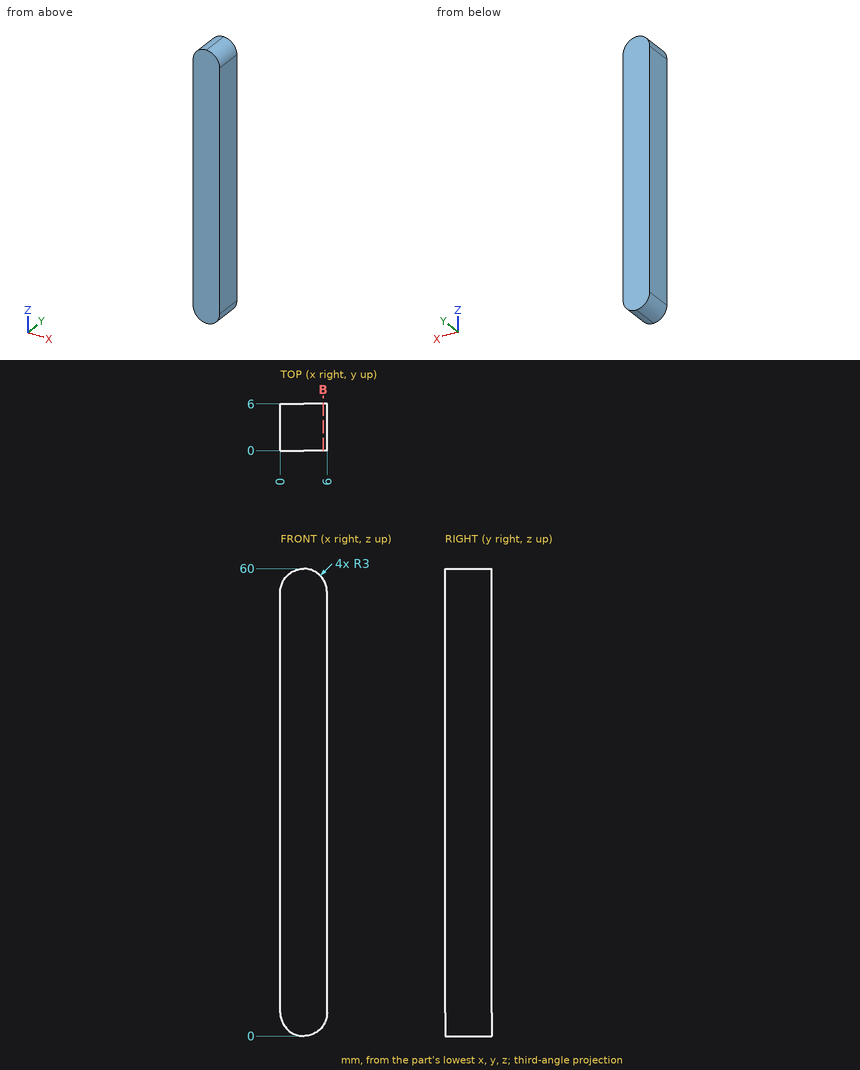
Could you check a few things on this drawing? It's one solid part, dimensions in mm from its lowest x, y, z. Coordinates: 2 decimals unless noted, no trailing zeros. Order: outer loops, then holes, each group sorted by start corner. A loop starts at its lowest first (then second) coordinate and runs counter-clockwise, first axis right, second up.
1) Imagine slicing it at B-B on x = 5.5. List the corners of the cut face in (y, z) for me, and give its area (3 significant figures).
2) I need wall thicknesses on line 1 (Z direction, x = 4.5, y = 3.4); line 2 (Z direction, x = 2, y = 1.6). Which ranges of each line are inside material? Lowest first, please.
3) Will this pin go through, and if not, where does the flat tip stop? pin 1 (1 mm diameter, centred on y = 3, z = 27, fed in from -X).
Response values:
1. outline: (0, 1.34) - (6, 1.34) - (6, 58.66) - (0, 58.66) - close
1. area: 344 mm2
2. line 1: z = 0.4 to 59.6
2. line 2: z = 0.17 to 59.83
3. pin 1: stops at x = 0
